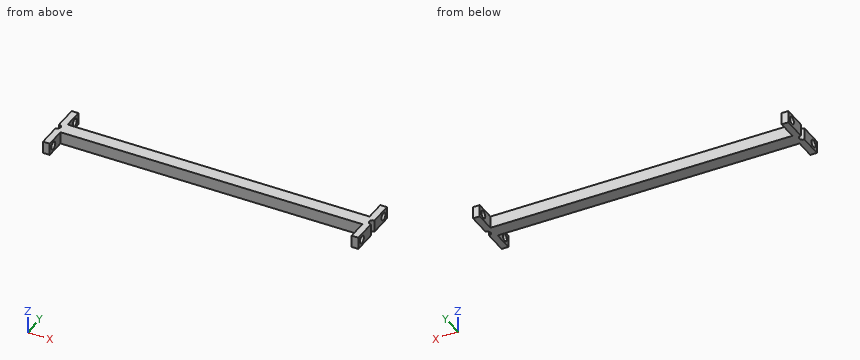
from build123d import *

# Parameters (mm, degrees)
SKETCH_1_W          = 235
SKETCH_1_H          = 10
EXTRUDE_1_DEPTH     = 9
SKETCH_2_W          = 5
SKETCH_2_H          = 40
EXTRUDE_2_DEPTH     = 9
SKETCH_3_R          = 2.5
CUT_EXTRUDE_1_DEPTH = 32
SKETCH_4_R          = 2.75
CUT_EXTRUDE_2_DEPTH = 237.497357279


with BuildPart() as part:
    # 草图1 → 凸台-拉伸1 (new body)
    with BuildSketch(Plane.XY):
        with Locations((117.5, -5)):
            Rectangle(SKETCH_1_W, SKETCH_1_H)
    extrude(amount=EXTRUDE_1_DEPTH)

    # 草图2 → 凸台-拉伸2 (add)
    with BuildSketch(Plane.XY.offset(9)):
        with Locations((232.5, -5)):
            Rectangle(SKETCH_2_W, SKETCH_2_H)
        with Locations((2.5, -5)):
            Rectangle(SKETCH_2_W, SKETCH_2_H)
    extrude(amount=-EXTRUDE_2_DEPTH)

    # 草图3 → 切除-拉伸1 (cut)
    with BuildSketch(Plane.XY.offset(9)):
        with Locations((235, -5)):
            Circle(SKETCH_3_R)
        with Locations((0, -5)):
            Circle(SKETCH_3_R)
    extrude(amount=-CUT_EXTRUDE_1_DEPTH, mode=Mode.SUBTRACT)

    # 草图4 → 切除-拉伸2 (cut, through all)
    with BuildSketch(Plane.ZY):
        with Locations(Location((4.5, 10, 0), (0, 0, 270))):
            Circle(SKETCH_4_R)
        with Locations(Location((4.5, -20, 0), (0, 0, 270))):
            Circle(SKETCH_4_R)
    extrude(amount=-CUT_EXTRUDE_2_DEPTH, mode=Mode.SUBTRACT)


solid = part.part
CAD build for the part. Positions are in the model's coordinates, mm. Round coordinates to 2 decimals unless told otherwise and drop trailing zeros. Write each loop counter-clockwise with the first axis right and the second up, starting at its lowest first coordinate (ties: lowest second). Pieces come first, ordered by that corner, then holes. Notation, with made-up numbers: M 10,-35 L 22,-35 A22 cw 22,-7 Z; hole C -30,38 d6. An arc over 180 degrees is marked long. Put each result on its own line as item: value. Start each with the question number.
1) Pin check, flat tips, straight feed: pin 1 Ø2.5 at (y, z) = (7.5, 5.5) entering from -X; pin 2 Ø4 at (x, z) = (132, 8) entering from +Y; pin 3 Ø2 at (x, z) = (90, 8) entering from -Y; pin 4 Ø2 at (y, z) = (-4, 2) entering from +X. Stop position of each tip, or through.
2) Saw through at A-A, the plane y = -14.5. Write the cut outline in (x, z), and give its area (3 significant figures).
3) Saw through at D-D, the plane x = 42.5. Write the cut outline in (y, z), and give its area (3 significant figures).
4) Saw through at C-C, the plane y = 10. Write the cut outline in (x, z), and give its area (3 significant figures).
5) Drill centre lines: probe 1 along Z at (x, y) = (232.55, -20); probe 2 along X at (y, z) = (-14, 4.5); probe 3 along Y at (x, z) = (211, 7.75). Where is each one in solid material? Low to high. Write a range as [from, to].
6) Saw through at B-B, the plane z = 4.5. Count the separate pieces of the cut face and the enclosed holes in it, and give its area (3 significant figures).
Resolved:
1. pin 1: x = 0
1. pin 2: y = 0
1. pin 3: y = -10
1. pin 4: x = 233.5
2. outline: M 0,0 L 5,0 L 5,9 L 0,9 Z; M 230,0 L 235,0 L 235,9 L 230,9 Z
2. area: 90.0 mm²
3. outline: M -10,0 L 0,0 L 0,9 L -10,9 Z
3. area: 90.0 mm²
4. outline: M 0,0 L 5,0 L 5,1.75 L 0,1.75 Z; M 0,7.25 L 5,7.25 L 5,9 L 0,9 Z; M 230,0 L 235,0 L 235,1.75 L 230,1.75 Z; M 230,7.25 L 235,7.25 L 235,9 L 230,9 Z
4. area: 35.0 mm²
5. probe 1: [0, 1.75], [7.25, 9]
5. probe 2: [0, 5], [230, 235]
5. probe 3: [-10, 0]
6. separate pieces: 5
6. enclosed holes: 0
6. area: 2,520 mm²
